For this review, take the finished solid that the model builds, in its own axes (mm). A direction names the side the tool comes from. Round coordinates to 2 decimals unless told otherwise and drop trailing zeros. Order: outer loops, then holes, each group sorted by start corner. A loop starts at its lowest first (then second) coordinate and runs counter-clockwise, first axis right, second up. Notation, with made-up numbers: M 60,71.25 L 119,71.25 A8 ccw 119,79.25 Z; hole C 41.25,-16 d3. An arc over 180 degrees is marked long. Use a Markdown table: item, result.
from build123d import *

# Parameters (mm, degrees)
ESQUISSE1_R                  = 1
BOSS_EXTRU_1_DEPTH           = 3.5
BOSS_EXTRU_1_DEPTH_BACK      = 11
ESQUISSE2_R                  = 2
BOSS_EXTRU_2_DEPTH           = 2
ESQUISSE3_OUTSIDE_W          = 9.488
ESQUISSE3_OUTSIDE_H          = 9.488
ENL_V_MAT_EXTRU_1_DEPTH      = 1
ENL_V_MAT_EXTRU_1_DEPTH_BACK = 17.5
CHANFREIN1_SIZE              = 0.5
ESQUISSE4_R                  = 1
ENL_V_MAT_EXTRU_2_DEPTH      = 5.5


with BuildPart() as part:
    # Esquisse1 → Boss.-Extru.1 (new body, two sides)
    with BuildSketch(Plane.XY) as boss_extru_1_sk:
        with Locations((2.7, 1.35)):
            Circle(ESQUISSE1_R)
    extrude(amount=BOSS_EXTRU_1_DEPTH)
    extrude(boss_extru_1_sk.sketch, amount=-BOSS_EXTRU_1_DEPTH_BACK)

    # Esquisse2 → Boss.-Extru.2 (add)
    with BuildSketch(Plane.XY.offset(3.5)):
        with Locations((2.7, 1.35)):
            Circle(ESQUISSE2_R)
    extrude(amount=BOSS_EXTRU_2_DEPTH)

    # Esquisse3 outside → Enlèv. mat.-Extru.1 (cut, two sides)
    with BuildSketch(Plane.XY.offset(5.5)) as enl_v_mat_extru_1_sk:
        with Locations((2.7, 1.35)):
            Rectangle(ESQUISSE3_OUTSIDE_W, ESQUISSE3_OUTSIDE_H)
        with BuildLine():
            Line((1.4, 2.869868415), (1.4, 0.05))
            Line((1.4, 0.05), (4, 0.05))
            Line((4, 0.05), (4, 2.869868415))
            ThreePointArc((4, 2.869868415), (2.7, 3.35), (1.4, 2.869868415))
        make_face(mode=Mode.SUBTRACT)
    extrude(amount=ENL_V_MAT_EXTRU_1_DEPTH, mode=Mode.SUBTRACT)
    extrude(enl_v_mat_extru_1_sk.sketch, amount=-ENL_V_MAT_EXTRU_1_DEPTH_BACK, mode=Mode.SUBTRACT)

    # Chanfrein1
    chanfrein1_edges = [part.edges().sort_by_distance(p)[0] for p in [
        (2.7, 0.05, 5.5),
    ]]
    chamfer(chanfrein1_edges, length=CHANFREIN1_SIZE)

    # Esquisse4 → Enlèv. mat.-Extru.2 (cut)
    with BuildSketch(Plane(origin=(0, 0, -11), x_dir=(-1, 0, 0), z_dir=(0, 0, -1))):
        with Locations((-2.7, 1.35)):
            Circle(ESQUISSE4_R)
    extrude(amount=-ENL_V_MAT_EXTRU_2_DEPTH, mode=Mode.SUBTRACT)


solid = part.part
Q1. Add section D-D (x = 3.25). Write out the cut boundary in (y, z).
Determined:
| item | result |
|---|---|
| outline | M 0.05,3.5 L 0.51,3.5 L 0.51,-5.5 L 2.19,-5.5 L 2.19,3.5 L 3.27,3.5 L 3.27,5.5 L 0.55,5.5 L 0.05,5 Z |
Q2. Add section B-B (x = 2.7). Write out the cut boundary in (y, z).
Determined:
| item | result |
|---|---|
| outline | M 0.05,3.5 L 0.35,3.5 L 0.35,-5.5 L 2.35,-5.5 L 2.35,3.5 L 3.35,3.5 L 3.35,5.5 L 0.55,5.5 L 0.05,5 Z |
Q3. Add section C-C (z = -4.5). Write out the cut boundary in (x, y).
Determined:
| item | result |
|---|---|
| outline | C 2.7,1.35 d2 |
Q4. Machinability: for faces 1 (the flat face through (2.4, 2.5, 3.5)), 2 (the flat face through (4, 1, 5)), which of the approach directions +Z, -Z, +X, -X, +Y, -Y give a long, thin tool a straight path to every point of the face, cutting with its end or side? Answer none if there is none.
Determined:
| item | result |
|---|---|
| face 1 | -Z |
| face 2 | +Z, -Z, +X, +Y, -Y |
Q5. Add section A-A (y = 1.35). Write out the cut boundary in (x, z), then the cut area to 3 significant figures.
Determined:
| item | result |
|---|---|
| outline | M 1.4,3.5 L 1.7,3.5 L 1.7,-5.5 L 3.7,-5.5 L 3.7,3.5 L 4,3.5 L 4,5.5 L 1.4,5.5 Z |
| area | 23.2 mm^2 |
Q6. Wall thickness on line 1 along Z through (x, y) = (1.6, 2.6); line 2 along Y through (x, z) = (2.65, -3.5); line 3 along Z through (x, y) = (2.25, 0.35): over which ranges is each line inside the solid? List them lowest first. Write a range as [from, to].
Determined:
| item | result |
|---|---|
| line 1 | z = [3.5, 5.5] |
| line 2 | y = [0.35, 2.35] |
| line 3 | z = [3.5, 5.3] |
